Verification items for the finished model (mm, model axes). Face numbers are marked on the shaded views. A direction names the side the tool comes from. Give positions to 0.01 mm unless a question says otherwise; leave off trailing zeros. Write each loop counter-clockwise with the first axis right and the second up, starting at its lowest first coordinate (ties: lowest second). Pieces come first, ordered by that corner, then holes. Notation, with made-up numbers: (-1.5, 74.25) -> (51.5, 74.25) arc R4 cw to (51.5, 81.25) -> close; hole circle Ø7 at (-17.75, -36). An arc over 180 degrees is marked (long way). Answer as CSV lines item,"result".
Autodesk Inventor part; units mm, degrees
ref_plane "Work Plane1" through (0, 0, 3.81) normal (0, 0, -1) x (-1, 0, 0)
ref_plane "YZ Plane" through (0, 0, 0) normal (1, 0, 0) x (0, 1, 0)
ref_plane "XZ Plane" through (0, 0, 0) normal (0, 1, 0) x (-1, 0, 0)
sketch "Sketch1" plane through (0, 0, 0) normal (0, 0, 1) x (1, 0, 0)
  circle A0 centre (0, 0) radius 19.05
  dimension "d0" = 38.1
extrude "wheel" add sketch "Sketch1" along normal blind 7.62
sketch "Sketch2" plane through (0, 0, 7.62) normal (0, 0, 1) x (1, 0, 0)
  circle A0 centre (0, 0) radius 19.05
  circle A1 centre (0, 0) radius 3.81
  dimension "d4" = 7.62
extrude "axle" add sketch "Sketch2" along normal blind 5.08 and the other way blind 12.7 contours A1
sketch "Sketch3" plane through (0, 0, 12.7) normal (0, 0, 1) x (1, 0, 0)
  line L0 (-11.1125, -17.4625) -> (28.575, -17.4625)
  line L1 (28.575, -17.4625) -> (28.575, 17.4625)
  line L2 (28.575, 17.4625) -> (-11.1125, 17.4625)
  line L3 (-17.4625, 11.1125) -> (-17.4625, -11.1125)
  arc A0 (-11.1125, 17.4625) -> (-17.4625, 11.1125) centre (-11.1125, 11.1125) ccw
  arc A1 (-17.4625, -11.1125) -> (-11.1125, -17.4625) centre (-11.1125, -11.1125) ccw
  point P0 (-17.4625, -17.4625)
  point P1 (-17.4625, 17.4625)
  dimension "d13" = 6.35
extrude "side" add sketch "Sketch3" against normal blind 1.524
ref_plane "Work Plane1" through (0, 0, 3.81) normal (0, 0, -1) x (-1, 0, 0)
mirror "Mirror1" about plane through (0, 0, 3.81) normal (0, 0, -1) of "side"
sketch "Sketch4" plane through (28.575, -17.4625, 12.7) normal (1, 0, 0) x (0, 0, -1)
  line L0 (0, 0) -> (18.1871, 0)
  line L1 (18.1871, 0) -> (18.1871, 34.925)
  line L2 (18.1871, 34.925) -> (0, 34.925)
  line L3 (0, 34.925) -> (0, 0)
  point P0 (12.7, 17.4625)
extrude "Extrusion4" add sketch "Sketch4" along normal blind 1.524
sketch "Sketch5" plane through (30.099, -17.4625, 12.7) normal (1, 0, 0) x (0, 0, -1)
  line L0 (0, 0) -> (18.1871, 0)
  line L1 (18.1871, 34.925) -> (0, 34.925)
  line L2 (8.0841, 6.35) -> (10.103, 6.35)
  line L3 (10.103, 6.35) -> (10.103, 25.4)
  line L4 (10.103, 25.4) -> (8.0841, 25.4)
  line L5 (8.0841, 25.4) -> (8.0841, 6.35)
  line L6 (9.0935, 34.925) -> (9.0935, 0) construction
  line L7 (9.0935, 25.4) -> (9.0935, 6.35) construction
  point P0 (12.7, 17.4625)
extrude "Extrusion5" add sketch "Sketch5" along normal blind 25.4
sketch "Sketch6" plane through (30.099, -11.1125, 4.6159) normal (0, 0, 1) x (1, 0, 0)
  line L0 (25.4, 19.05) -> (25.4, 0)
  circle A0 centre (12.7, 9.525) radius 4.7625
  point P0 (-30.099, 11.1125)
  dimension "d19" = 12.7
extrude "Extrusion6" cut sketch "Sketch6" against normal blind 25.4
properties part number "0pulley" material "Steel, Alloy"
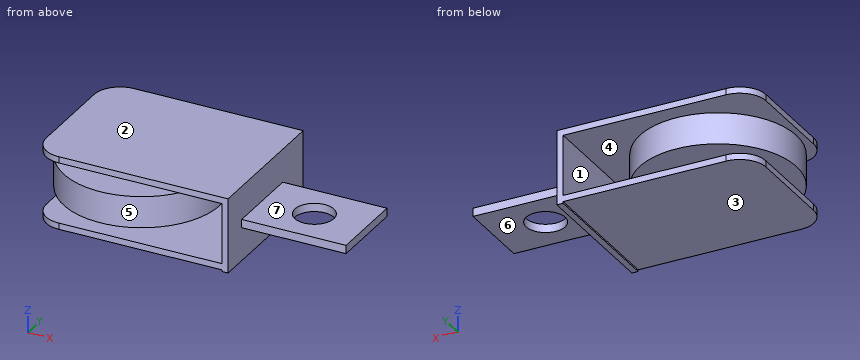
1) Scan lines: line 1 along Z through (x, y) = (22.5, -4.5); line 2 along X through (y, z) = (-2, 2.75) (3 decimals); line 3 along Z through (x, y) = (-9.5, -15.5). Record each from-to range of solid material in increasing order.
Reported:
line 1,"-5.08 to -3.56, 11.18 to 12.7"
line 2,"-18.945 to 18.945, 28.575 to 38.054, 47.544 to 55.499"
line 3,"-5.08 to -3.56, 0 to 7.62, 11.18 to 12.7"
2) Draft check along Z on the marked faces 4, 5, 6 and 7. Enter one of: +Z half, -Z half, draft (parallel to the pull), parting line (faces both ways), or undercut.
Reported:
face 4,"undercut"
face 5,"undercut"
face 6,"-Z half"
face 7,"+Z half"
3) Section check A-A (x = 27.5). Record the boundary of the cut face in (y, z).
Reported:
outline,"(-17.46, -5.08) -> (17.46, -5.08) -> (17.46, -3.56) -> (-17.46, -3.56) -> close; (-17.46, 11.18) -> (17.46, 11.18) -> (17.46, 12.7) -> (-17.46, 12.7) -> close"
4) Section check D-D (y = -8.5). Record the boundary of the cut face in (x, z) (1 decimal), and give its area (3 significant figures).
Reported:
outline,"(-17.5, -5.1) -> (28.6, -5.1) -> (28.6, -5.5) -> (30.1, -5.5) -> (30.1, 2.6) -> (55.5, 2.6) -> (55.5, 4.6) -> (30.1, 4.6) -> (30.1, 12.7) -> (-17.5, 12.7) -> (-17.5, 11.2) -> (28.6, 11.2) -> (28.6, -3.6) -> (-17.5, -3.6) -> close; (-17, 0) -> (17, 0) -> (17, 7.6) -> (-17, 7.6) -> close"
area,"479 mm²"
5) Tool access check on the marked faces 1, 2 and 3. Record the directions out of +Z, -Z, +X, -X, +Y, -Y that give a thin tool (end or side, any length) a straight path to the whole face; none if there is none.
Reported:
face 1,"+Y, -Y"
face 2,"+Z, +X, -X, +Y, -Y"
face 3,"-Z, -X, +Y, -Y"
6) Section check B-B (y = 0). State how many separate pieces and enclosed holes the cut face has, and give its area (3 significant figures).
Reported:
separate pieces,"2"
enclosed holes,"1"
area,"546 mm²"
7) Depth check by flat-ended pin: pin 1 (11.5 mm diameter, centred on x = 2.5, y = 7, fed in from -Z); pin 2 (5.5 mm diameter, centred on x = 41.5, y = -4.5, fed in from +Z); pin 3 (15 mm diameter, centred on x = 45, y = -0.5, fed in from -Z). Enter the tip coordinate at first touch or a pass-through.
Reported:
pin 1,"z = -5.08"
pin 2,"z = 4.62"
pin 3,"z = 2.6"
